Geometry check sheet. Reference: the model listing, model coordinates, mm. Face numbers are marked on the shaded views. A direction names the side the tool comes from. Round coordinates to 2 decimals unless told otherwise and drop trailing zeros. Loops run counter-clockwise (first coordinate to the right, second up) from the corner with the lowest first, then second, coordinate; pieces in that order, holes last.
```python
from build123d import *

# Parameters (mm, degrees)
F0_W     = 40
F0_H     = 19.3
F1_DEPTH = 3
F0_H_2   = 2
F2_DEPTH = 5.6
F3_W     = 40
F3_H     = 5.3
F4_DEPTH = 3.2
F5_R     = 1
F3_H_2   = 1.8
F6_DEPTH = 1.4


with BuildPart() as f1:
    # F0 (on Top) → F1 (new body)
    with BuildSketch(Plane.XY):
        with Locations((20, -11.65)):
            Rectangle(F0_W, F0_H)
    extrude(amount=F1_DEPTH)

    # F0 (on Top) → F2 (join)
    with BuildSketch(Plane.XY):
        with Locations((20, -22.3)):
            Rectangle(F0_W, F0_H_2)
        with Locations((20, -1)):
            Rectangle(F0_W, F0_H_2)
    extrude(amount=F2_DEPTH)

    # F0 (on Top) + F3 (on Top) → F4 (join)
    with BuildSketch(Plane.XY):
        with Locations((20, -1)):
            Rectangle(F0_W, F0_H_2)
    with BuildSketch(Plane.XY):
        with Locations((20, -20.65)):
            Rectangle(F3_W, F3_H)
    extrude(amount=-F4_DEPTH)

    # F5
    f5_edges = [f1.edges().sort_by_distance(p)[0] for p in [
        (20, -23.3, -3.2),
        (20, 0, -3.2),
    ]]
    fillet(f5_edges, radius=F5_R)

    # F3 (on Top) → F6 (join)
    with BuildSketch(Plane.XY):
        with Locations((20, -9.1)):
            Rectangle(F3_W, F3_H_2)
        with Locations((20, -10.9)):
            Rectangle(F3_W, F3_H_2)
    extrude(amount=-F6_DEPTH)


solid = f1.part
```
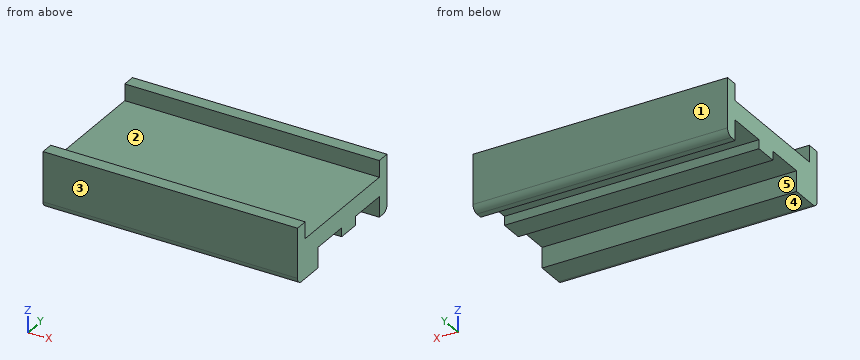
1) Mould release check, pull along Y, two halves, no side actions. Record for the marked faces 1, 2 and 3: +Y half, -Y half, draft (parallel to the pull), parting line (faces both ways), or undercut.
Report:
face 1: +Y half
face 2: undercut
face 3: -Y half
2) Sectioned sample at D-D, the plane y = -15.5. Record the cut outline in (x, z), then the cut area to 3 significant figures.
Report:
outline: (0, 0) - (40, 0) - (40, 3) - (0, 3) - close
area: 120 mm2
3) Scan lines: line 1 along Y through (x, z) = (11.5, -1.25); line 2 along Y through (x, z) = (10, 5); line 3 along Y through (x, z) = (28, -1.75). Record each from-to range of solid material in increasing order.
Report:
line 1: y = -23.3 to -18, -11.8 to -8.2, -2 to 0
line 2: y = -23.3 to -21.3, -2 to 0
line 3: y = -23.3 to -18, -2 to 0
4) Access from +Z, -Z, +X, -X, +Y, -Y to the whole of each face (thin tool, end or side, straight path). Record for the marked faces 4 and 5.
Report:
face 4: -Z, +X, -X, +Y, -Y
face 5: -Z, +X, -X
5) Sectioned sample at B-B, the plane z = 3.5. Record the cut outline in (x, y).
Report:
outline: (0, -23.3) - (40, -23.3) - (40, -21.3) - (0, -21.3) - close; (0, -2) - (40, -2) - (40, 0) - (0, 0) - close
6) Sectioned sample at A-A, the plane z = -0.75. Record the cut outline in (x, y), then the cut area to 3 significant figures.
Report:
outline: (0, -23.3) - (40, -23.3) - (40, -18) - (0, -18) - close; (0, -11.8) - (40, -11.8) - (40, -8.2) - (0, -8.2) - close; (0, -2) - (40, -2) - (40, 0) - (0, 0) - close
area: 436 mm2
7) Sectioned sample at C-C, the plane x = 16.5. Record the cut outline in (y, z).
Report:
outline: (-23.3, -2.2) arc R1 ccw to (-22.3, -3.2) - (-18, -3.2) - (-18, 0) - (-11.8, 0) - (-11.8, -1.4) - (-8.2, -1.4) - (-8.2, 0) - (-2, 0) - (-2, -3.2) - (-1, -3.2) arc R1 ccw to (0, -2.2) - (0, 5.6) - (-2, 5.6) - (-2, 3) - (-21.3, 3) - (-21.3, 5.6) - (-23.3, 5.6) - close
8) Gauge pin test, flat ends, axial feed: pin 1 (6 mm diameter, centred on x = 14, y = -17, fed in from +Z); pin 2 (5 mm diameter, centred on x = 17, y = -14, fed in from -Z). Record the tip position at first contact, or that the pin passes through.
Report:
pin 1: stops at z = 3
pin 2: stops at z = -1.4
